Here's how the part is built. I have some questions about the finished solid (model axes, mm). Give positions to 0.01 mm unless a question says otherwise; leave off trailing zeros. Loops run counter-clockwise (first coordinate to the right, second up) from the corner with the lowest first, then second, coordinate; pieces in that order, holes last.
Q1. Suppose I cut it at B-B (z = 0.85). List the corners of the cut face in (x, y) for me.
Q2. Suppose I cut it at D-D (x = -129.5). List the corners of the cut face in (y, z) for me, and give its area (3 significant figures).
Q3. Suppose I cut it at A-A (x = -86). List the corners of the cut face in (y, z) for me.
Q4. Suppose I cut it at C-C (y = -270). List the corners of the cut face in (x, z) for me, and give its area (3 significant figures).
Q5. I'm going to push flat-ended pins straight in: P1, Ø1, axis at x = -62.5, z = 1.5, coming from the +Y side; P2, Ø1, axis at x = -61.5, z = 1, coming from the -Y side; P3, Ø1, axis at y = -226.5, z = 1.5, coming from the +X side. Where does each tip first touch, or does it pass through?
Q6. I need wall thicknesses on probe 1 along Y at (x, z) = (-150, 0.7); probe 2 along Y at (x, z) = (-140, 1.4); probe 3 along X at (y, z) = (-284, 0.3). Which ranges of each line are inside material? Lowest first, please.
```python
from build123d import *

# Parameters (mm, degrees)
SKETCH1_W           = 17.080006479
SKETCH1_H           = 20.0800081
BOSS_EXTRUDE1_DEPTH = 2


with BuildPart() as part:
    # Sketch1 → Boss-Extrude1 (new body)
    with BuildSketch(Plane.XY):
        Polygon((-158.225691519, -298.776294453), (-158.225691519, -313.236290403), (-149.725691519, -313.236290403), (-149.725691519, -321.736290403), (-66.725691519, -321.736290403), (-66.725691519, -313.236290403), (-58.225691519, -313.236290403), (-58.225691519, -230.236290403), (-66.725691519, -230.236290403), (-66.725691519, -221.736290403), (-149.725691519, -221.736290403), (-149.725691519, -230.236290403), (-158.225691519, -230.236290403), (-158.225691519, -278.696286353), (-137.765694759, -278.696286353), (-137.765694759, -261.696286353), (-120.68568828, -261.696286353), (-120.68568828, -277.85605527), (-108.863916488, -277.85605527), (-108.863916488, -281.776294453), (-108.863916488, -298.776294453), (-122.185689089, -298.776294453), align=None)
        with Locations((-87.225691519, -271.736290403)):
            Rectangle(SKETCH1_W, SKETCH1_H, mode=Mode.SUBTRACT)
    extrude(amount=BOSS_EXTRUDE1_DEPTH)


solid = part.part
```
Solutions:
1. outline: (-158.23, -313.24) - (-149.73, -313.24) - (-149.73, -321.74) - (-66.73, -321.74) - (-66.73, -313.24) - (-58.23, -313.24) - (-58.23, -230.24) - (-66.73, -230.24) - (-66.73, -221.74) - (-149.73, -221.74) - (-149.73, -230.24) - (-158.23, -230.24) - (-158.23, -278.7) - (-137.77, -278.7) - (-137.77, -261.7) - (-120.69, -261.7) - (-120.69, -277.86) - (-108.86, -277.86) - (-108.86, -298.78) - (-158.23, -298.78) - close; hole (-95.77, -281.78) - (-78.69, -281.78) - (-78.69, -261.7) - (-95.77, -261.7) - close
2. outline: (-321.74, 0) - (-298.78, 0) - (-298.78, 2) - (-321.74, 2) - close; (-261.7, 0) - (-221.74, 0) - (-221.74, 2) - (-261.7, 2) - close
2. area: 126 mm2
3. outline: (-321.74, 0) - (-281.78, 0) - (-281.78, 2) - (-321.74, 2) - close; (-261.7, 0) - (-221.74, 0) - (-221.74, 2) - (-261.7, 2) - close
4. outline: (-158.23, 0) - (-137.77, 0) - (-137.77, 2) - (-158.23, 2) - close; (-120.69, 0) - (-95.77, 0) - (-95.77, 2) - (-120.69, 2) - close; (-78.69, 0) - (-58.23, 0) - (-58.23, 2) - (-78.69, 2) - close
4. area: 132 mm2
5. P1: stops at y = -230.24
5. P2: stops at y = -313.24
5. P3: stops at x = -66.73
6. probe 1: y = -313.24 to -298.78, -278.7 to -230.24
6. probe 2: y = -321.74 to -298.78, -278.7 to -221.74
6. probe 3: x = -108.86 to -58.23
